from build123d import *

# Parameters (mm, degrees)
CYLINDER1792_R         = 74
CYLINDER1792_DEPTH     = 60
BOX754_W               = 80
BOX754_H               = 6
BOX754_DEPTH           = 20
BOX754_PLACEMENT_ANGLE = 71.4
BOX752_W               = 44
BOX752_H               = 6
BOX752_DEPTH           = 49


with BuildPart() as obj1:
    # Cylinder1792 → Cylinder1792 (new body)
    with BuildSketch(Plane.XY.offset(26)):
        Circle(CYLINDER1792_R)
    extrude(amount=CYLINDER1792_DEPTH)


with BuildPart() as krychle754:
    # Box754 → Box754 (new body)
    with BuildSketch(Plane.XY):
        with Locations((40, 3)):
            Rectangle(BOX754_W, BOX754_H)
    extrude(amount=BOX754_DEPTH)


with BuildPart() as krychle754_1:
    # Box754 placement: moved
    add(krychle754.part.moved(Location((-118.17, -24, 82.63))).rotate(Axis((-118.17, -24, 82.63), (0, 1, 0)), BOX754_PLACEMENT_ANGLE))


with BuildPart() as cut555:
    # Box752 → Box752 (new body)
    with BuildSketch(Plane(origin=(-93, -24, 29), x_dir=(1, 0, 0), z_dir=(0, 0, 1))):
        with Locations((22, 3)):
            Rectangle(BOX752_W, BOX752_H)
    extrude(amount=BOX752_DEPTH)

    # Cut548: cut Krychle754
    add(krychle754_1.part, mode=Mode.SUBTRACT)

    # Cut555: cut obj1
    add(obj1.part, mode=Mode.SUBTRACT)


solid = cut555.part
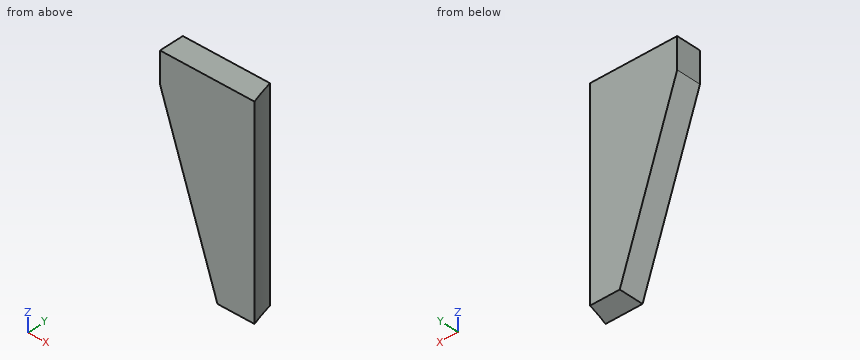
Read the model definition and answer for the solid it produces. Units are mm, in the model's axes. Round coordinates to 2 decimals unless told otherwise and drop trailing zeros. Order: outer loops, then holes, each group sorted by start corner. A loop starts at its lowest first (then second) coordinate and runs counter-clockwise, first axis right, second up. Notation, with made-up numbers: (-32.75, 81) - (-8.75, 81) arc R27 cw to (-8.75, 103) - close; hole circle Ø7 at (64.5, 13.25). An arc over 180 degrees is marked (long way). Use one line per item in the form item = value. Start each with the question number.
(1) The part is cut by section B-B (x = -83). Give the vertices of the cut face in (y, z), then the cut area to 3 significant figures.
(2) The part is cut by section C-C (z = 54). Give the vertices of the cut face in (x, y), then the cut area to 3 significant figures.
(3) The part is cut by section A-A (y = -22.75). Give the vertices of the cut face in (x, z), then the cut area to 3 significant figures.
(4) The part is cut by section D-D (y = -19). Give the vertices of the cut face in (x, z), then the cut area to 3 significant figures.
(5) Find the intervals of material crossed by line 1 along X through (y, z) = (-19, 47); line 2 along X through (y, z) = (-20.75, 62.5), in increasing order. Write a range as from..to.
Checked values:
q1.outline = (-24, 40.83) - (-18, 40.83) - (-18, 78) - (-24, 78) - close
q1.area = 223 mm^2
q2.outline = (-87.43, -24) - (-70, -24) arc R74 cw to (-71.78, -18) - (-87.43, -18) - close
q2.area = 99.0 mm^2
q3.outline = (-93, 70.54) - (-79.02, 29) - (-70.42, 29) - (-70.42, 78) - (-93, 78) - close
q3.area = 816 mm^2
q4.outline = (-93, 70.54) - (-79.02, 29) - (-71.52, 29) - (-71.52, 78) - (-93, 78) - close
q4.area = 762 mm^2
q5.line_1 = -85.08..-71.52
q5.line_2 = -90.29..-71.03
